```python
from build123d import *

# Parameters (mm, degrees)
SKETCH1_R      = 2.975
EXTRUDE1_DEPTH = 0.575
SKETCH2_R      = 2.47
EXTRUDE2_DEPTH = 7.55
FILLET2_R      = 2.47
SKETCH4_W      = 13.081078865
SKETCH4_H      = 5.810496129
EXTRUDE3_DEPTH = 0.36
SKETCH5_W      = 0.5
SKETCH5_H      = 0.5
EXTRUDE4_DEPTH = 20
SKETCH6_W      = 0.5
SKETCH6_H      = 0.5
EXTRUDE5_DEPTH = 4


with BuildPart() as part:
    # Sketch1 → Extrude1 (new, symmetric)
    with BuildSketch(Plane.XY):
        Circle(SKETCH1_R)
    extrude(amount=EXTRUDE1_DEPTH, both=True)

    # Sketch2 → Extrude2 (add)
    with BuildSketch(Plane.XY.offset(0.575)):
        Circle(SKETCH2_R)
    extrude(amount=EXTRUDE2_DEPTH)

    # Fillet2
    fillet2_edges = [part.edges().sort_by_distance(p)[0] for p in [
        (-2.47, 0, 8.125),
    ]]
    fillet(fillet2_edges, radius=FILLET2_R)

    # Sketch4 → Extrude3 (cut)
    with BuildSketch(Plane(origin=(0, 3, 0), x_dir=(-1, 0, 0), z_dir=(0, 1, 0))):
        with Locations((-1.941605697, 0.17278636)):
            Rectangle(SKETCH4_W, SKETCH4_H)
    extrude(amount=-EXTRUDE3_DEPTH, mode=Mode.SUBTRACT)

    # Sketch5 → Extrude4 (add)
    with BuildSketch(Plane(origin=(0, 0, -0.575), x_dir=(-1, 0, 0), z_dir=(0, 0, -1))):
        with Locations((0, 1.26)):
            Rectangle(SKETCH5_W, SKETCH5_H)
        with Locations((0, -1.26)):
            Rectangle(SKETCH5_W, SKETCH5_H)
    extrude(amount=EXTRUDE4_DEPTH)

    # Sketch6 → Extrude5 (cut)
    with BuildSketch(Plane(origin=(0, 0, -20.575), x_dir=(-1, 0, 0), z_dir=(0, 0, -1))):
        with Locations((0, 1.26)):
            Rectangle(SKETCH6_W, SKETCH6_H)
    extrude(amount=-EXTRUDE5_DEPTH, mode=Mode.SUBTRACT)


solid = part.part
```
Work out the finished part from the listing and answer in its coordinate system (mm). A direction names the side the tool comes from. Give positions to 0.01 mm unless a question says otherwise; leave off trailing zeros. Order: outer loops, then holes, each group sorted by start corner. A loop starts at its lowest first (then second) coordinate and runs counter-clockwise, first axis right, second up. Notation, with made-up numbers: M 41.25,-39 L 82.25,-39 A24 ccw 82.25,-18 Z; hole C -10.75,17.5 d11. An arc over 180 degrees is marked long. Return JSON: item names as keys, results as strings.
1) Each of these flat-tipped pins is pushed along its axis until it touches: pin 1 (0.6 mm diameter, centred on y = -1.5, z = -9.5, fed in from -X); pin 2 (0.6 mm diameter, centred on x = 0, y = 1.5, fed in from -Z) (3 decimals); pin 3 (3 mm diameter, centred on y = -2.5, z = -13, fed in from +X); pin 4 (3 mm diameter, centred on x = 1, y = 0.5, fed in from +Z) (3 decimals). Where does it stop, or does it pass through?
Resolved:
{"pin 1": "x = -0.25", "pin 2": "z = -16.575", "pin 3": "x = 0.25", "pin 4": "z = 8.125"}
2) Straight lines are drawn through the part: line 1 along X through (y, z) = (1.1, -11.5); line 2 along Z through (x, y) = (-2.7, 0.2) (3 decimals); line 3 along Y through (x, z) = (-0.85, 2.25). For each, find the intervals that lie inside material, in ascending order. Write a range as [from, to].
Resolved:
{"line 1": "[-0.25, 0.25]", "line 2": "[-0.575, 0.575]", "line 3": "[-2.32, 2.32]"}
3) Section D-D, the plane z = 2.75 is taken. Write down the section's boundary in (x, y), plus the area to 3 significant figures.
Resolved:
{"outline": "C 0,0 d4.94", "area": "19.2 mm^2"}
4) Section A-A, the plane z = -15.25 is taken. Write down the section's boundary in (x, y), plus the area to 3 significant figures.
Resolved:
{"outline": "M -0.25,-1.51 L 0.25,-1.51 L 0.25,-1.01 L -0.25,-1.01 Z; M -0.25,1.01 L 0.25,1.01 L 0.25,1.51 L -0.25,1.51 Z", "area": "0.500 mm^2"}
5) Section C-C, the plane y = 0 is taken. Write down the section's boundary in (x, z) (3 decimals), plus the area to 3 significant figures.
Resolved:
{"outline": "M -2.975,-0.575 L 2.975,-0.575 L 2.975,0.575 L 2.47,0.575 L 2.47,5.655 A2.47 ccw -2.47,5.655 L -2.47,0.575 L -2.975,0.575 Z", "area": "41.5 mm^2"}
6) A tool of negligible diameter and unlimited length cuts with its end or side. For faces 1 (the cylindrical face through (2.356, 0.742, 3.079)), 2 (the flat face through (0, 2.64, 0)), from which of +Z, -Z, +X, -X, +Y, -Y can it reach the whole face along a straight path? Write none if from no direction.
Resolved:
{"face 1": "+Z", "face 2": "+Z, -Z, +X, -X, +Y"}
7) Section B-B, the plane x = 0 is taken. Write down the section's boundary in (y, z) (3 decimals), plus the area to 3 significant figures.
Resolved:
{"outline": "M -2.975,-0.575 L -1.51,-0.575 L -1.51,-20.575 L -1.01,-20.575 L -1.01,-0.575 L 1.01,-0.575 L 1.01,-16.575 L 1.51,-16.575 L 1.51,-0.575 L 2.64,-0.575 L 2.64,0.575 L 2.47,0.575 L 2.47,5.655 A2.47 ccw -2.47,5.655 L -2.47,0.575 L -2.975,0.575 Z", "area": "59.1 mm^2"}
